The listing builds one solid part. Answer for the finished solid, in the listing's coordinates (mm). Face numbers are marked on the shaded views. A direction names the side the tool comes from. Give positions to 0.01 mm unless a question says otherwise; leave off trailing zeros. Write each loop counter-clockwise with the first axis right and the second up, starting at its lowest first coordinate (ties: lowest second). Pieces come first, ordered by that corner, then holes. Notation, with made-up numbers: (-29.75, 18) -> (20.25, 18) arc R14 ccw to (20.25, 26) -> close; hole circle Ø8 at (46.5, 33). An arc over 180 degrees is marked (long way). Write each question's results on one line, items separated by ' | '. Start each with the question number.
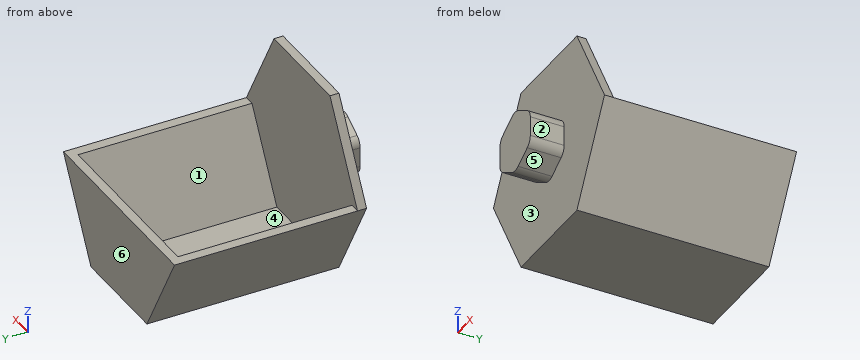
from build123d import *

# Parameters (mm, degrees)
F1_DEPTH = 4
F3_DEPTH = 15
F4_R     = 5
F6_DEPTH = 85
F8_DEPTH = 4


with BuildPart() as f1:
    # F0 (on Front) → F1 (new body)
    with BuildSketch(Plane.XZ):
        Polygon((-22.6691420217, 40.6), (0, 0), (23, 0), (46, 0), (68.6691420217, 40.6), (46, 81.2), (0, 81.2), align=None)
    extrude(amount=F1_DEPTH)

    # F2 (on face) → F3 (join)
    with BuildSketch(Plane.XZ.offset(4)):
        with BuildLine():
            ThreePointArc((29.2500001164, 29.7746825199), (33.8253175809, 34.3500000582), (35.5, 40.6))
            ThreePointArc((35.5, 40.6), (33.8253175809, 46.8499999418), (29.2500001164, 51.4253174801))
            ThreePointArc((29.2500001164, 51.4253174801), (23, 53.1), (16.7499998836, 51.4253174801))
            ThreePointArc((16.7499998836, 51.4253174801), (12.1746824191, 46.8499999418), (10.5, 40.6))
            ThreePointArc((10.5, 40.6), (12.1746825605, 34.3499998133), (16.7500003734, 29.7746822371))
            ThreePointArc((16.7500003734, 29.7746822371), (23.0000002828, 28.1), (29.2500001164, 29.7746825199))
        make_face()
        with BuildLine():
            Line((35.5, 33.3831216351), (35.5, 40.6))
            ThreePointArc((35.5, 40.6), (33.8253175809, 34.3500000582), (29.2500001164, 29.7746825199))
            Line((29.2500001164, 29.7746825199), (35.5, 33.3831216351))
        make_face()
        with BuildLine():
            ThreePointArc((29.2500001164, 51.4253174801), (33.8253175809, 46.8499999418), (35.5, 40.6))
            Line((35.5, 40.6), (35.5, 47.8168783649))
            Line((35.5, 47.8168783649), (29.2500001164, 51.4253174801))
        make_face()
        with BuildLine():
            ThreePointArc((16.7499998836, 51.4253174801), (23, 53.1), (29.2500001164, 51.4253174801))
            Line((29.2500001164, 51.4253174801), (23, 55.0337567297))
            Line((23, 55.0337567297), (16.7499998836, 51.4253174801))
        make_face()
        with BuildLine():
            Line((23, 26.1662432703), (29.2500001164, 29.7746825199))
            ThreePointArc((29.2500001164, 29.7746825199), (23.0000002828, 28.1), (16.7500003734, 29.7746822371))
            Line((16.7500003734, 29.7746822371), (23, 26.1662432703))
        make_face()
        with BuildLine():
            ThreePointArc((10.5, 40.6), (12.1746824191, 46.8499999418), (16.7499998836, 51.4253174801))
            Line((16.7499998836, 51.4253174801), (10.5, 47.8168783649))
            Line((10.5, 47.8168783649), (10.5, 40.6))
        make_face()
        with BuildLine():
            Line((10.5, 33.3831216351), (16.7500003734, 29.7746822371))
            ThreePointArc((16.7500003734, 29.7746822371), (12.1746825605, 34.3499998133), (10.5, 40.6))
            Line((10.5, 40.6), (10.5, 33.3831216351))
        make_face()
    extrude(amount=F3_DEPTH)

    # F4
    f4_edges = [f1.edges().sort_by_distance(p)[0] for p in [
        (35.5, -11.5, 47.816878),
        (23, -11.5, 55.033757),
        (10.5, -11.5, 47.816878),
        (35.5, -11.5, 33.383122),
        (23, -11.5, 26.166243),
        (10.5, -11.5, 33.383122),
    ]]
    fillet(f4_edges, radius=F4_R)

    # F5 (on face) → F6 (join)
    with BuildSketch(Plane.XZ.offset(4)):
        Polygon((64.0878597141, 40.6), (43.6521314402, 4.0000013266), (2.3478685598, 4.0000013266), (-18.0878597141, 40.6), (-22.6691420217, 40.6), (0, 0), (46, 0), (68.6691420217, 40.6), align=None)
    extrude(amount=-F6_DEPTH)

    # F7 (on face) → F8 (join)
    with BuildSketch(Plane(origin=(0, 81, 0), x_dir=(-1, 0, 0), z_dir=(0, 1, 0))):
        Polygon((22.6691420217, 40.6), (-68.6691420217, 40.6), (-46, 0), (0, 0), align=None)
    extrude(amount=-F8_DEPTH)


solid = f1.part
1. Section D-D (z = 42) is taken. Write down the section's boundary in (x, y), then the cut area to 3 significant figures.
2. The mould has two halves that part along Y. Classify the marked faces 4, 5 and 6: pulls with the +Y half, pulls with the -Y half, needs draft (parallel to the pull), parting line crosses it, or undercut.
3. Section C-C (x = 29) is taken. Write down the section's boundary in (y, z).
4. Each of these flat-tipped pins is pushed along its axis until it touches: pin 1 Ø1 at (y, z) = (67.5, 26.5) entering from -X; pin 2 Ø10 at (y, z) = (-0.5, 24.5) entering from -X; pin 3 Ø7 at (y, z) = (-14.5, 40) entering from +X. Where does it stop, or does it pass through?
5. A tool of negligible diameter and unlimited length cuts with its end or side. For the marked faces 1, 2 and 3, from which of +Z, -Z, +X, -X, +Y, -Y can it reach the whole face along a straight path? Write none if from no direction.
6. Section A-A (z = 20.5) is taken. Write down the section's boundary in (x, y), then the cut area to 3 significant figures.
7. Section B-B (y = 28) is taken. Write down the section's boundary in (x, z).
8. Consider probe 1 along Y at (x, z) = (63.5, 40); probe 2 along Z at (x, y) = (11, 27.5); probe 3 along Y at (x, z) = (-5, 16.5). Determine where each line is inside the solid, lowest interval first. Write a range as [from, to].
Results:
1) outline: (-21.89, -4) -> (10.5, -4) -> (10.5, -19) -> (35.5, -19) -> (35.5, -4) -> (67.89, -4) -> (67.89, 0) -> (-21.89, 0) -> close | area: 734 mm²
2) face 4: undercut | face 5: needs draft | face 6: pulls with the +Y half
3) outline: (-19, 29.63) -> (-4, 29.63) -> (-4, 0) -> (81, 0) -> (81, 40.6) -> (77, 40.6) -> (77, 4) -> (0, 4) -> (0, 81.2) -> (-4, 81.2) -> (-4, 51.57) -> (-19, 51.57) -> close
4) pin 1: stops at x = -15.08 | pin 2: stops at x = -16.47 | pin 3: stops at x = 35.5
5) face 1: +Z | face 2: +Z, -Z, +X, -Y | face 3: -Y
6) outline: (-11.45, -4) -> (57.45, -4) -> (57.45, 81) -> (-11.45, 81) -> close; hole (-6.86, 0) -> (52.86, 0) -> (52.86, 77) -> (-6.86, 77) -> close | area: 1,260 mm²
7) outline: (-22.67, 40.6) -> (0, 0) -> (46, 0) -> (68.67, 40.6) -> (64.09, 40.6) -> (43.65, 4) -> (2.35, 4) -> (-18.09, 40.6) -> close
8) probe 1: y = [-4, 0], [77, 81] | probe 2: z = [0, 4] | probe 3: y = [-4, 81]
